Design review of the part built by this model. Coordinates are the model's own, in mm. Face numbers are marked on the shaded views. A direction names the side the tool comes from. Give positions to 0.01 mm unless a question says otherwise; leave off trailing zeros. Order: outer loops, then holes, each group sorted by start corner. A loop starts at its lowest first (then second) coordinate and runs counter-clockwise, first axis right, second up. Notation, with made-up numbers: (58, 4.5) -> (117, 4.5) arc R17 ccw to (117, 32.5) -> close; hole circle Ø3 at (-27, 35.25). An arc over 180 degrees is marked (long way). One line per item, written item: value.
from build123d import *

# Parameters (mm, degrees)
EXTRUDE_1_DEPTH     = 5
CUT_EXTRUDE_1_DEPTH = 3
CUT_EXTRUDE_2_DEPTH = 6.5


with BuildPart() as part:
    # Эскиз1 → Бобышка-Вытянуть1 (new body, symmetric)
    with BuildSketch(Plane.XY):
        Polygon((5, 0), (-5, 0), (-5, -3), (-9.75, -3), (-9.75, -8.5), (9.75, -8.5), (9.75, -3), (5, -3), align=None)
    extrude(amount=EXTRUDE_1_DEPTH, both=True)

    # Эскиз3 → Отверстие обработанное метчиком M62 (revolve, cut)
    with BuildSketch(Plane(origin=(0, 0, 0), x_dir=(0, 0, 1), z_dir=(1, 0, 0))):
        Polygon((0, 0), (0, 8.5), (3.5, 8.5), (2.5, 7.5), (2.5, 1), (3.5, 0), align=None)
    revolve(axis=Axis((0, 6.35, 0), (0, -1, 0)), mode=Mode.SUBTRACT)

    # Эскиз4 → Вырез-Вытянуть1 (cut)
    with BuildSketch(Plane(origin=(0, 0, 0), x_dir=(1, 0, 0), z_dir=(0, 1, 0))):
        with BuildLine():
            Line((-5, 5), (-5, 0))
            ThreePointArc((-5, 0), (-3.535533906, 3.535533906), (0, 5))
            Line((0, 5), (-5, 5))
        make_face()
        with BuildLine():
            Line((0, -5), (5, -5))
            Line((5, -5), (5, 0))
            ThreePointArc((5, 0), (3.535533906, -3.535533906), (0, -5))
        make_face()
    extrude(amount=-CUT_EXTRUDE_1_DEPTH, mode=Mode.SUBTRACT)

    # Эскиз5 → Вырез-Вытянуть2 (cut, through all)
    with BuildSketch(Plane(origin=(0, -3, 0), x_dir=(1, 0, 0), z_dir=(0, 1, 0))):
        with BuildLine():
            Line((-9.75, 0), (-9.75, 5))
            Line((-9.75, 5), (-8.370334521, 5))
            ThreePointArc((-8.370334521, 5), (-9.398756875, 2.59342808), (-9.75, 0))
        make_face()
        with BuildLine():
            Line((9.75, 0), (9.75, -5))
            Line((9.75, -5), (8.370334521, -5))
            ThreePointArc((8.370334521, -5), (9.398756875, -2.59342808), (9.75, 0))
        make_face()
    extrude(amount=-CUT_EXTRUDE_2_DEPTH, mode=Mode.SUBTRACT)

    # Вырез-По траектории1: sweep along a path in Эскиз7
    with BuildLine(Plane.XZ.offset(8.5)) as sweep_1_path:
        Line((0, 9.75), (-9.75, 9.75))
        Line((-9.75, 9.75), (-9.75, 0))
        ThreePointArc((-9.75, 0), (-6.894291117, -6.894291117), (0, -9.75))
        Line((0, -9.75), (9.75, -9.75))
        Line((9.75, -9.75), (9.75, 0))
        ThreePointArc((9.75, 0), (6.894291117, 6.894291117), (0, 9.75))
    # Эскиз6 → Вырез-По траектории1 (sweep, cut)
    with BuildSketch(Plane.XY.offset(5)):
        Polygon((-9.75, -5.5), (-9.75, -8.5), (-5, -8.5), align=None)
    sweep(path=sweep_1_path.line, transition=Transition.RIGHT, mode=Mode.SUBTRACT)


solid = part.part
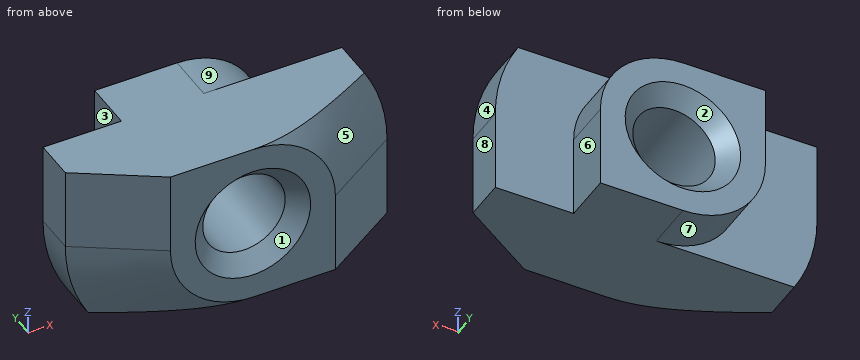
Item 1: Add section B-B on y = -2. Give the boundary of the cut face in (x, z), plus the area to 3 significant figures.
Returned:
outline: (-5, 0) arc R5 ccw to (0, -5) -> (5, -5) -> (5, 0) arc R5 ccw to (0, 5) -> (-5, 5) -> close; hole circle Ø5 at (0, 0)
area: 69.6 mm²
Item 2: Machinability: for the marked faces 5, 6, 7, 8 and 9, which of the approach directions +Z, -Z, +X, -X, +Y, -Y give a long, thin tool a straight path to every point of the face, cutting with its end or side? Answer none if there is none.
Returned:
face 5: +Z, +X, -Y
face 6: +Z, -Z, +X, +Y
face 7: -Z, -X, +Y
face 8: +Z, -Z, +X, +Y, -Y
face 9: +Z, +X, +Y
Item 3: Draft analysis for pull direction Z (two halves, no side actions). For the marked faces 1, 2, 3 and 4, state which applies: pulls with the +Z half, pulls with the -Z half, needs draft (parallel to the pull), parting line crosses it, or undercut.
Returned:
face 1: undercut
face 2: undercut
face 3: needs draft
face 4: pulls with the +Z half
Item 4: Add section A-A on y = -4.5. Give the boundary of the cut face in (x, z), plus the area to 3 significant figures.
Returned:
outline: (-9.75, 0) arc R9.75 ccw to (-8.37, -5) -> (9.75, -5) -> (9.75, 0) arc R9.75 ccw to (8.37, 5) -> (-9.75, 5) -> close; hole circle Ø5 at (0, 0)
area: 171 mm²
Item 5: Clearance check with flat-ended pins moving along their axes: P1, Ø1.5, axis at y = -1.5, z = 1.5, coming from the -X side; P2, Ø2, axis at y = -1, z = -1.5, coming from the +X side; P3, Ø5, axis at y = -4, z = 4, coming from the +X side. State where each tip first meets the part, or that it passes through.
Returned:
P1: x = -5
P2: x = 5
P3: x = 9.63
Item 6: To check wall thickness, follow line 1 along Z through (x, y) = (0, -4.25); line 2 along Z through (x, y) = (-2, -2.75). State the ranges of each line that lie inside material, in increasing order. Write a range as from..to.
Returned:
line 1: -5..-2.5, 2.5..5
line 2: -4.58..-1.5, 1.5..5
